CAD build for the part. Positions are in the model's coordinates, mm. Face numbers are marked on the shaded views. Coordinates: 2 decimals unless noted, no trailing zeros. Write each loop counter-clockwise with the first axis right and the second up, starting at its lowest first coordinate (ties: lowest second). Pieces come first, ordered by that corner, then holes. Notation, with made-up numbers: (-35, 73) -> (-5, 73) arc R23 cw to (-5, 106) -> close; hole circle Ø6 at (68, 26.25). An arc over 180 degrees is marked (long way). Answer as CSV lines item,"result".
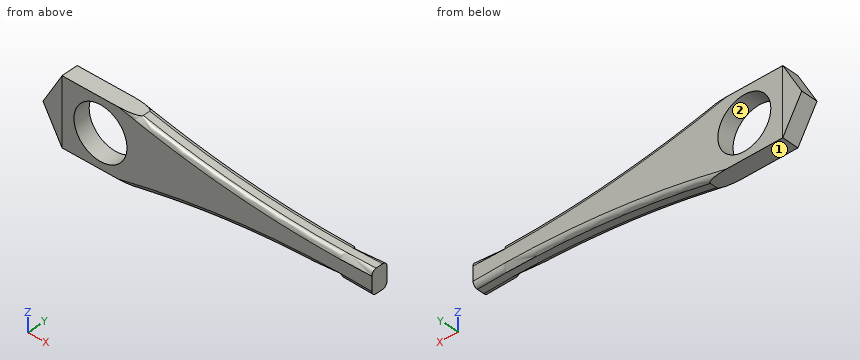
Autodesk Inventor part; units mm, degrees
ref_plane "YZ Plane" through (0, 0, 0) normal (1, 0, 0) x (0, 1, 0)
ref_plane "XZ Plane" through (0, 0, 0) normal (0, 1, 0) x (-1, 0, 0)
ref_plane "XY Plane" through (0, 0, 0) normal (0, 0, 1) x (1, 0, 0)
sketch "Sketch1" plane through (0, 0, 0) normal (0, 1, 0) x (-1, 0, 0)
  circle A0 centre (0, 0) radius 11.125
  line L0 (0, -11.125) -> (0, -14.125)
  line L1 (0, 11.125) -> (0, 14.125)
  line L2 (11.125, 0) -> (16.125, 0)
  line L3 (16.125, 14.125) -> (-113.875, 14.125)
  line L4 (-113.875, 14.125) -> (-113.875, -14.125)
  line L5 (-113.875, -14.125) -> (16.125, -14.125)
  line L6 (16.125, -14.125) -> (16.125, 14.125)
  dimension "d0" = 22.25
  dimension "d1" = 3
  dimension "d2" = 3
  dimension "d3" = 5
  dimension "d6" = 130
extrude "Extrusion1" add sketch "Sketch1" along normal blind 7 contours L2 L6 L5 L0 A0 | A0 L1 L3 L6 L2 | A0 L0 L5 L4 L3 L1
sketch "Sketch2" plane through (0, 0, 0) normal (0, -1, 0) x (1, 0, 0)
  line L0 (113.875, 14.125) -> (113.875, -14.125)
  line L1 (113.875, 0) -> (113.875, 5)
  line L2 (113.875, 5) -> (113.875, -5)
  circle A0 centre (0, 0) radius 11.125
  line L3 (11.125, 0) -> (16.125, 0)
  line L4 (-16.125, 14.125) -> (113.875, 14.125)
  line L5 (16.125, 14.125) -> (16.125, -14.125)
  line L6 (113.875, -14.125) -> (-16.125, -14.125)
  arc A1 (16.125, 14.125) -> (113.875, 5) centre (100.0237, 384.7475) ccw
  arc A2 (113.875, -5) -> (16.125, -14.125) centre (100.0237, -384.7475) ccw
  line L7 (16.125, 14.125) -> (113.875, 14.125)
  line L8 (113.875, 14.125) -> (113.875, 5)
  line L9 (16.125, -14.125) -> (113.875, -14.125)
  line L10 (113.875, -14.125) -> (113.875, -5)
  dimension "d9" = 5
  dimension "d10" = 10
  dimension "d11" = 5
  dimension "d12" = 380
  dimension "d13" = 380
extrude "Extrusion2" cut sketch "Sketch2" against normal through all contours L0 A1 L4 | L0 L6 A2
fillet "Fillet1" radius 2 1 edges at (64.7041, 0, 6.3924)
fillet "Fillet2" radius 2 1 edges at (64.7041, 7, 6.3924)
fillet "Fillet3" radius 2 1 edges at (64.7041, 0, -6.3924)
fillet "Fillet4" radius 2 1 edges at (64.7041, 7, -6.3924)
sketch "Sketch3" plane through (0, 0, 0) normal (0, -1, 0) x (1, 0, 0)
  line L0 (-16.125, -14.125) -> (-16.125, 14.125)
  line L1 (-16.125, 0) -> (-24.125, 0)
  line L2 (-24.125, 0) -> (-16.125, 14.125)
  line L3 (-16.125, 14.125) -> (-16.125, -14.125)
  line L4 (-16.125, -14.125) -> (-24.125, 0)
  point P0 (0, 0)
  dimension "d20" = 8
extrude "Extrusion3" add sketch "Sketch3" against normal blind 7
properties part number "Leg"
Item 1: Two-plate mould, pull along Z, no slides. Class the marked faces 1 and 2: pulls with the +Z half, pulls with the -Z half, needs draft (parallel to the pull), parting line crosses it, or undercut.
Answer below:
face 1,"pulls with the -Z half"
face 2,"undercut"
Item 2: Wall check: line 1 (Z direction, x = 0, y = 5.75) (3 decimals); line 2 (X direction, y = 3.5, z = 0) (3 decimals); line 3 (X direction, y = 5.25, z = -0.5) (3 decimals). Give the ranges that are in metal, low to high. Write a range as from..to.
Answer below:
line 1,"z = -14.125..-11.125, 11.125..14.125"
line 2,"x = -24.125..-11.125, 11.125..113.875"
line 3,"x = -23.842..-11.114, 11.114..113.875"
Item 3: Flat gauge pins, fed straight in: pin 1 (3 mm diameter, centred on x = 40, y = 5.5, fed in from +Z); pin 2 (1.5 mm diameter, centred on x = 63.5, y = 3.5, fed in from +Z). Where does each tip first touch, or does it go through?
Answer below:
pin 1,"stops at z = 9.75"
pin 2,"stops at z = 6.58"
Item 4: Saw through at A-A on x = 0. Give the cut face in (y, z) (3 decimals), and give its area (3 significant figures).
Answer below:
outline,"(0, -14.125) -> (7, -14.125) -> (7, -11.125) -> (0, -11.125) -> close; (0, 11.125) -> (7, 11.125) -> (7, 14.125) -> (0, 14.125) -> close"
area,"42.0 mm2"
